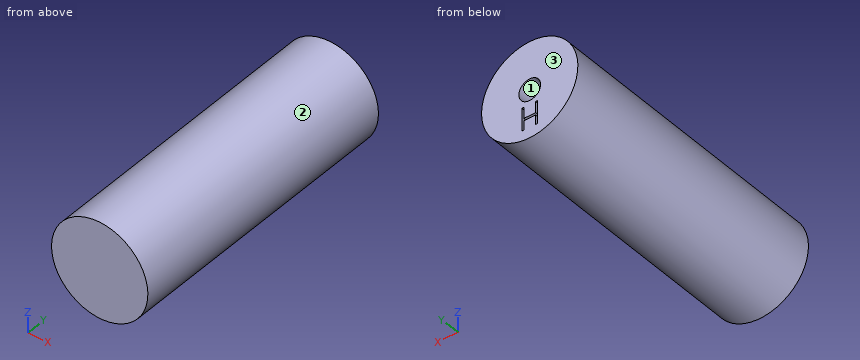
```python
from build123d import *

# Parameters (mm, degrees)
SKETCH1_R           = 10
BOSS_EXTRUDE1_DEPTH = 4
SKETCH2_R           = 10
SKETCH2_R_2         = 8
SKETCH2_R_3         = 3.5
BOSS_EXTRUDE2_DEPTH = 52
SKETCH3_R           = 10
BOSS_EXTRUDE3_DEPTH = 4
CUT_EXTRUDE1_DEPTH  = 2
SKETCH5_R           = 2.25
CUT_EXTRUDE2_DEPTH  = 50


with BuildPart() as part:
    # Sketch1 → Boss-Extrude1 (new body)
    with BuildSketch(Plane(origin=(0, 0, 0), x_dir=(1, 0, 0), z_dir=(0, 1, 0))):
        with Locations(Location((0, 0, 0), (0, 0, 270))):
            Circle(SKETCH1_R)
    extrude(amount=BOSS_EXTRUDE1_DEPTH)

    # Sketch2 → Boss-Extrude2 (add)
    # profile 1 of 2: a face of its own
    with BuildSketch(Plane(origin=(0, 4, 0), x_dir=(1, 0, 0), z_dir=(0, 1, 0))):
        with Locations(Location((0, 0, 0), (0, 0, 270))):
            Circle(SKETCH2_R)
        with Locations(Location((0, 0, 0), (0, 0, 90))):
            Circle(SKETCH2_R_2, mode=Mode.SUBTRACT)
    # profile 2 of 2: a face of its own
    with BuildSketch(Plane(origin=(0, 4, 0), x_dir=(1, 0, 0), z_dir=(0, 1, 0))):
        with Locations(Location((0, 0, 0), (0, 0, 90))):
            Circle(SKETCH2_R_3)
    extrude(amount=BOSS_EXTRUDE2_DEPTH)

    # Sketch3 → Boss-Extrude3 (add)
    with BuildSketch(Plane(origin=(0, 56, 0), x_dir=(1, 0, 0), z_dir=(0, 1, 0))):
        with Locations(Location((0, 0, 0), (0, 0, 270))):
            Circle(SKETCH3_R)
    extrude(amount=BOSS_EXTRUDE3_DEPTH)

    # Sketch4 → Cut-Extrude1 (cut)
    with BuildSketch(Plane(origin=(0, 60, 0), x_dir=(1, 0, 0), z_dir=(0, 1, 0))):
        Polygon((-1.648557692, 7.80697224), (-1.221153846, 7.80697224), (-1.221153846, 5.853126086), (1.221153846, 5.853126086), (1.221153846, 7.80697224), (1.648557692, 7.80697224), (1.648557692, 3.04447224), (1.221153846, 3.04447224), (1.221153846, 5.364664548), (-1.221153846, 5.364664548), (-1.221153846, 3.04447224), (-1.648557692, 3.04447224), align=None)
    extrude(amount=-CUT_EXTRUDE1_DEPTH, mode=Mode.SUBTRACT)

    # Sketch5 → Cut-Extrude2 (cut)
    with BuildSketch(Plane(origin=(0, 60, 0), x_dir=(1, 0, 0), z_dir=(0, 1, 0))):
        with Locations(Location((0, 0, 0), (0, 0, 270))):
            Circle(SKETCH5_R)
    extrude(amount=-CUT_EXTRUDE2_DEPTH, mode=Mode.SUBTRACT)


solid = part.part
```
Could you check a few things on this model? Use its own coordinates, in mm. Face numbers are marked on the shaded views. Give positions to 0.01 mm unless a question says otherwise; leave off trailing zeros. Write each loop counter-clockwise with the first axis right and the second up, starting at its lowest first coordinate (ties: lowest second). Pieces come first, ordered by that corner, then holes. Notation, with made-up numbers: (-5, 30.25) - (-1, 30.25) arc R18 ccw to (-1, 65.25) - close; hole circle Ø4 at (64.25, 49.5). An arc over 180 degrees is marked (long way). One line per item, written item: value. Start each with the question number.
Item 1: Imagine slicing it at D-D, the plane x = -5.75. List the corners of the cut face in (y, z) for me.
Item 2: Imagine slicing it at B-B, the plane x = 0. List the corners of the cut face in (y, z) for me, and give its area (3 significant figures).
Item 3: Please list where these lines run through material, in increasing order: line 1 (X direction, y = 39, z = 0); line 2 (Y direction, x = -7, z = 2); line 3 (Z direction, x = 2.5, y = 18.5). Write a range as from..to.
Item 4: I'm going to push flat-ended pins straight in: pin 1 (10 mm diameter, centred on x = 2, y = 20.5, fed in from +Z); pin 2 (10 mm diameter, centred on y = 33.5, z = -6, fed in from +X); pin 3 (1.5 mm diameter, centred on y = 52, z = -7.5, fed in from +X); pin 4 (0.6 mm diameter, centred on y = 59.5, z = -5, fed in from -X). Where does each tip first touch, or does it pass through?
Item 5: Imagine slicing it at A-A, the plane z = 0. List the corners of the cut face in (x, y) for me, and give its area (3 significant figures).
Item 6: Imagine slicing it at C-C, the plane y = 15.5. List the corners of the cut face in (x, z) for me.
Item 7: If we mould it in two halves opening along X, with no side actions, what happens to the marked faces 1, 2 and 3? For each: +X half, -X half, draft (parallel to the pull), parting line (faces both ways), or undercut.
Geometry says:
1. outline: (0, -8.18) - (60, -8.18) - (60, 8.18) - (0, 8.18) - close; hole (4, -5.56) - (56, -5.56) - (56, 5.56) - (4, 5.56) - close
2. outline: (0, -10) - (60, -10) - (60, -5.85) - (58, -5.85) - (58, -5.36) - (60, -5.36) - (60, -2.25) - (10, -2.25) - (10, 2.25) - (60, 2.25) - (60, 10) - (0, 10) - close; hole (4, -8) - (56, -8) - (56, -3.5) - (4, -3.5) - close; hole (4, 3.5) - (56, 3.5) - (56, 8) - (4, 8) - close
2. area: 506 mm^2
3. line 1: -10..-8, -3.5..-2.25, 2.25..3.5, 8..10
3. line 2: 0..4, 56..60
3. line 3: -9.68..-7.6, -2.45..2.45, 7.6..9.68
4. pin 1: z = 10
4. pin 2: x = 9.95
4. pin 3: x = 7.38
4. pin 4: x = -8.83
5. outline: (-10, 0) - (10, 0) - (10, 60) - (2.25, 60) - (2.25, 10) - (-2.25, 10) - (-2.25, 60) - (-10, 60) - close; hole (-8, 4) - (-3.5, 4) - (-3.5, 56) - (-8, 56) - close; hole (3.5, 4) - (8, 4) - (8, 56) - (3.5, 56) - close
5. area: 507 mm^2
6. outline: circle Ø20 at (0, 0); circle Ø7 at (0, 0); hole circle Ø16 at (0, 0); hole circle Ø4.5 at (0, 0)
7. face 1: undercut
7. face 2: parting line
7. face 3: draft
